Design review of the part built by this model. Coordinates are the model's own, in mm. Coordinates: 2 decimals unless noted, no trailing zeros. Write each loop counter-clockwise with the first axis right and the second up, starting at its lowest first coordinate (ties: lowest second). Pieces come first, ordered by that corner, then holes. Notation, with made-up numbers: (41, 86.5) - (55, 86.5) arc R28 cw to (55, 109.5) - close; hole circle Ø1 at (76, 10). An arc over 180 degrees is marked (long way). One line per item, written item: value.
from build123d import *

# Parameters (mm, degrees)
SKETCH1_W           = 195
SKETCH1_H           = 136
SKETCH1_W_2         = 171
SKETCH1_H_2         = 112
SKETCH1_W_3         = 160
SKETCH1_H_3         = 96
SKETCH1_W_4         = 27
SKETCH1_H_4         = 3
BOSS_EXTRUDE1_DEPTH = 2
SKETCH1_3_W         = 195
SKETCH1_3_H         = 136
BOSS_EXTRUDE2_DEPTH = 2
SKETCH2_R           = 3.175
CUT_EXTRUDE1_DEPTH  = 119.938009064


with BuildPart() as part:
    # Sketch1 → Boss-Extrude1 (new body)
    # profile 1 of 3: a face of its own
    with BuildSketch(Plane.XY):
        Rectangle(SKETCH1_W, SKETCH1_H)
        Polygon((85.5, 56), (85.5, -56), (13.5, -56), (13.5, -59), (-13.5, -59), (-13.5, -56), (-85.5, -56), (-85.5, 56), align=None, mode=Mode.SUBTRACT)
    # profile 2 of 3: a face of its own
    with BuildSketch(Plane.XY):
        Rectangle(SKETCH1_W_2, SKETCH1_H_2)
        with Locations((0, 3)):
            Rectangle(SKETCH1_W_3, SKETCH1_H_3, mode=Mode.SUBTRACT)
    # profile 3 of 3: a face of its own
    with BuildSketch(Plane.XY):
        with Locations((0, -57.5)):
            Rectangle(SKETCH1_W_4, SKETCH1_H_4)
    extrude(amount=-BOSS_EXTRUDE1_DEPTH)

    # Sketch1_3 → Boss-Extrude2 (add)
    with BuildSketch(Plane.XY):
        Rectangle(SKETCH1_3_W, SKETCH1_3_H)
        Polygon((85.5, 56), (85.5, -56), (13.5, -56), (13.5, -59), (-13.5, -59), (-13.5, -56), (-85.5, -56), (-85.5, 56), align=None, mode=Mode.SUBTRACT)
    extrude(amount=BOSS_EXTRUDE2_DEPTH)

    # Sketch2 → Cut-Extrude1 (cut, through all)
    with BuildSketch(Plane.XY.offset(2)):
        with Locations((-92.5, 63)):
            Circle(SKETCH2_R)
        with Locations((0, 63)):
            Circle(SKETCH2_R)
        with Locations((92.5, 63)):
            Circle(SKETCH2_R)
        with Locations((92.5, -63)):
            Circle(SKETCH2_R)
        with Locations((0, -63)):
            Circle(SKETCH2_R)
        with Locations((-92.5, -63)):
            Circle(SKETCH2_R)
    extrude(amount=-CUT_EXTRUDE1_DEPTH, mode=Mode.SUBTRACT)


solid = part.part
1. Consider section A-A, the plane x = 0. Write out the cut boundary in (y, z) (3 decimals).
Answer block:
outline: (-68, -2) - (-66.175, -2) - (-66.175, 2) - (-68, 2) - close; (-59.825, -2) - (-45, -2) - (-45, 0) - (-59, 0) - (-59, 2) - (-59.825, 2) - close; (51, -2) - (59.825, -2) - (59.825, 2) - (56, 2) - (56, 0) - (51, 0) - close; (66.175, -2) - (68, -2) - (68, 2) - (66.175, 2) - close
2. Consider section D-D, the plane y = -63. Write out the cut boundary in (x, z) (3 decimals).
Answer block:
outline: (-97.5, -2) - (-95.675, -2) - (-95.675, 2) - (-97.5, 2) - close; (-89.325, -2) - (-3.175, -2) - (-3.175, 2) - (-89.325, 2) - close; (3.175, -2) - (89.325, -2) - (89.325, 2) - (3.175, 2) - close; (95.675, -2) - (97.5, -2) - (97.5, 2) - (95.675, 2) - close
3. Mouldability with a two-part tool opening along Y and no side actions: class faces 1 (the face through (-1, -68, 0)), 2 (the face through (-97.5, -1, 0)), 3 (the face through (1.707, 65.677, 0.028)) as released by +Y, released by -Y, zero draft, split by the parting line, or undercut.
Answer block:
face 1: released by -Y
face 2: zero draft
face 3: undercut
4. Consider section B-B, the plane y = 22.5. Write out the cut boundary in (x, z).
Answer block:
outline: (-97.5, -2) - (-80, -2) - (-80, 0) - (-85.5, 0) - (-85.5, 2) - (-97.5, 2) - close; (80, -2) - (97.5, -2) - (97.5, 2) - (85.5, 2) - (85.5, 0) - (80, 0) - close
5. Consider section C-C, the plane x = -92.5. Write out the cut boundary in (y, z) (3 decimals).
Answer block:
outline: (-68, -2) - (-66.175, -2) - (-66.175, 2) - (-68, 2) - close; (-59.825, -2) - (59.825, -2) - (59.825, 2) - (-59.825, 2) - close; (66.175, -2) - (68, -2) - (68, 2) - (66.175, 2) - close
6. Wall thickness on line 1 along Y through (x, z) = (-92.5, 1.1) (3 decimals); line 2 along X through (y, z) = (52, 1.1); line 3 along Y through (x, z) = (-4, -0.65): over which ranges is each line inside the solid? List them lowest first.
Answer block:
line 1: y = -68 to -66.175, -59.825 to 59.825, 66.175 to 68
line 2: x = -97.5 to -85.5, 85.5 to 97.5
line 3: y = -68 to -45, 51 to 68
